Autodesk Inventor part; units mm, degrees
ref_plane "YZ Plane" through (0, 0, 0) normal (1, 0, 0) x (0, 1, 0)
ref_plane "XZ Plane" through (0, 0, 0) normal (0, 1, 0) x (-1, 0, 0)
ref_plane "XY Plane" through (0, 0, 0) normal (0, 0, 1) x (1, 0, 0)
sketch "Sketch1" plane through (0, 0, 0) normal (1, 0, 0) x (0, 1, 0)
  line L0 (-3.6662, -6.35) -> (-7.3323, 0)
  line L1 (-7.3323, 0) -> (-3.6662, 6.35)
  line L2 (-3.6662, 6.35) -> (3.6662, 6.35)
  line L3 (3.6662, 6.35) -> (7.3323, 0)
  line L4 (7.3323, 0) -> (3.6662, -6.35)
  line L5 (3.6662, -6.35) -> (-3.6662, -6.35)
  point P0 (0, 0)
  point P1 (0, 0)
  dimension "d0" = 12.7
extrude "Extrusion1" add sketch "Sketch1" along normal blind 43.1038
sketch "Sketch2" plane through (43.1038, 0, 0) normal (1, 0, 0) x (0, 0, -1)
  circle A0 centre (0, 0) radius 2.5527
  dimension "d3" = 5.1054
extrude "Extrusion2" cut sketch "Sketch2" against normal blind 43.1038
properties part number "INDX_015_OuterHex" material "Aluminum 6061"
The listing builds one solid part. Answer for the finished solid, in the listing's coordinates (mm). Give positions to 0.01 mm unless a question says otherwise; leave off trailing zeros. Order: outer loops, then holes, each group sorted by start corner. A loop starts at its lowest first (then second) coordinate and runs counter-clockwise, first axis right, second up. Notation, with made-up numbers: (38.25, -21.75) -> (97.25, -21.75) arc R29 cw to (97.25, 17.25) -> close; hole circle Ø1 at (84.5, 18). An arc over 180 degrees is marked (long way). Answer as CSV lines item,"result". Start each with the question number.
Q1. Given pin 1 (4 mm diameter, centred on y = 0, z = 0, fed in from -X); pin 2 (1.5 mm diameter, centred on x = 4.5, z = -3.5, fed in from -Y); pin 3 (6 mm diameter, centred on x = 8, z = 4.5, fed in from -Y), each flat-ended and moving along its own axis, determine where each tip first touches the part or whether it passes through.
Q2. Find the intervals of material crossed by L1, parallel to Y at x = 10.5, z = 0; L2, parallel to Y at x = 22, z = 1; L3, parallel to Z at x = 34.5, y = 1, in increasing order.
Q3. Determine the mould class of faces 1 (the flat face through (21.25, -5.474, -3.219)), 2 (the flat face through (21.25, 5.525, -3.131)), 3 (the cylindrical face through (21.854, 0.767, -2.435)) for opening direction Y: pulls with the +Y half, pulls with the -Y half, needs draft (parallel to the pull), parting line crosses it, or undercut.
Q4. A cutting plane is placed at C-C (x = 6). Determine the outline of the cut face in (y, z), then the cut area to 3 significant figures.
Q5. A cutting plane is placed at D-D (z = 4.5). Determine the outline of the cut face in (x, y), then the cut area to 3 significant figures.
Q6. A cutting plane is placed at B-B (y = 0). Determine the outline of the cut face in (x, z).
Q7. A cutting plane is placed at A-A (z = 1.5). Determine the outline of the cut face in (x, y).
Results found:
1,pin 1,"through"
1,pin 2,"y = -5.74"
1,pin 3,"y = -6.47"
2,L1,"-7.33 to -2.55, 2.55 to 7.33"
2,L2,"-6.75 to -2.35, 2.35 to 6.75"
2,L3,"-6.35 to -2.35, 2.35 to 6.35"
3,face 1,"pulls with the -Y half"
3,face 2,"pulls with the +Y half"
3,face 3,"undercut"
4,outline,"(-7.33, 0) -> (-3.67, -6.35) -> (3.67, -6.35) -> (7.33, 0) -> (3.67, 6.35) -> (-3.67, 6.35) -> close; hole circle Ø5.11 at (0, 0)"
4,area,"119 mm2"
5,outline,"(0, -4.73) -> (43.1, -4.73) -> (43.1, 4.73) -> (0, 4.73) -> close"
5,area,"408 mm2"
6,outline,"(0, -6.35) -> (43.1, -6.35) -> (43.1, -2.55) -> (0, -2.55) -> close; (0, 2.55) -> (43.1, 2.55) -> (43.1, 6.35) -> (0, 6.35) -> close"
7,outline,"(0, -6.47) -> (43.1, -6.47) -> (43.1, -2.07) -> (0, -2.07) -> close; (0, 2.07) -> (43.1, 2.07) -> (43.1, 6.47) -> (0, 6.47) -> close"
